Check sheet for the drawn part. Datum: minimum x, y, z corner. Units: mm. Round coordinates to 2 decimals unless told otherwise and drop trailing zeros. Write each loop counter-clockwise with the first axis right and the second up, starting at its lowest first coordinate (ties: lowest second). Pieces come first, ordered by that corner, then holes. Notation, with made-up numbers: (69.5, -36.5) - (86.5, -36.5) arc R28 cw to (86.5, -12.5) - close; hole circle Ø4 at (49.25, 6.25). An arc over 180 degrees is marked (long way). Answer as a JSON object with one key per item and string values. Group by question number.
Item 1: Release check for a two-part mould opening along Y. For the marked faces 1, 2 and 3 record: pulls with the +Y half, pulls with the -Y half, needs draft (parallel to the pull), parting line crosses it, or undercut.
Item 2: Thickness scan on line 1 (Z direction, x = 61, y = 6.5); line 2 (Y direction, x = 50, z = 12.75); line 3 (Y direction, x = 50, z = 2.3). Record the ranges inside material, lowest first.
Item 3: Gauge pin test, flat ends, axial feed: P1, Ø3, axis at x = 18, z = 6.5, coming from the +Y side; P2, Ø12, axis at x = 38, z = 8.5, coming from the +Y side; P3, Ø2, axis at x = 16, y = 29, coming from the +Z side (3 decimals); P4, Ø2, axis at y = 15, z = 10, coming from the +X side. Record the tip position at first contact, or that the pin passes through.
Item 4: Sectioned sample at A-A on z = 17. Record the boundary of the cut face in (x, y).
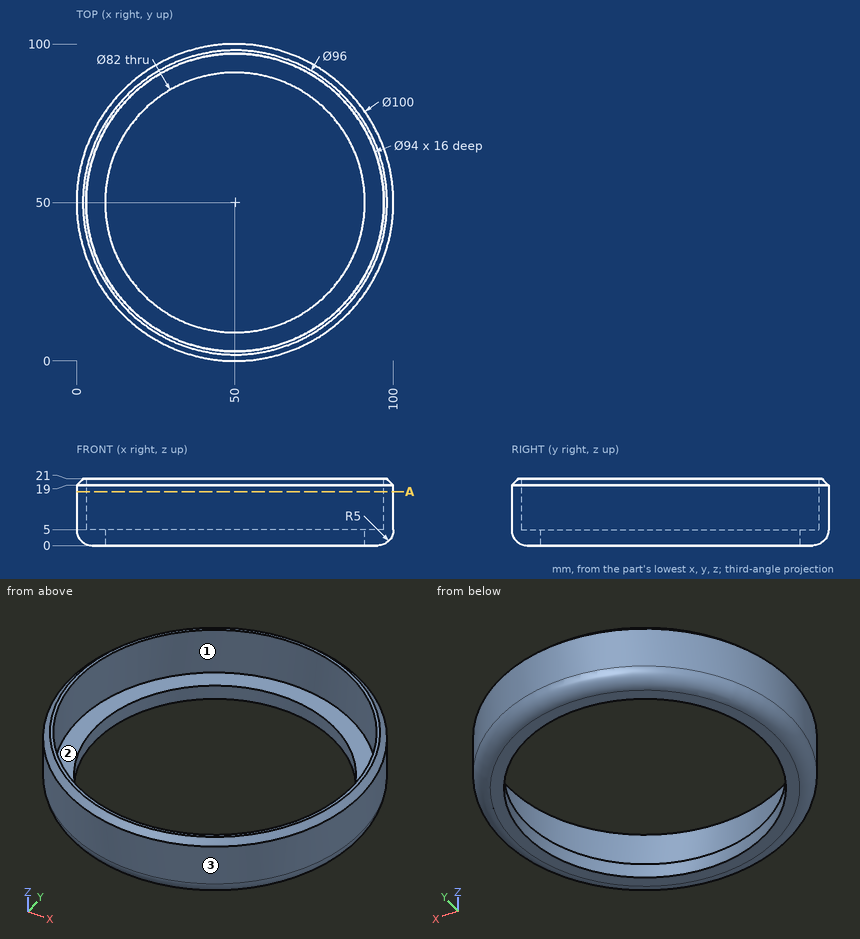
Completed:
{
 "1": {"face 1": "undercut", "face 2": "undercut", "face 3": "parting line crosses it"},
 "2": {"line 1": "0 to 5", "line 2": "0 to 3, 97 to 100", "line 3": "0.79 to 9, 91 to 99.21"},
 "3": {"P1": "y = 89.62", "P2": "y = 99.64", "P3": "through", "P4": "x = 86.66"},
 "4": {"outline": "circle Ø100 at (50, 50); hole circle Ø94 at (50, 50)"}
}
